Geometry check sheet. Reference: the model listing, model coordinates, mm. Coordinates: 2 decimals unless noted, no trailing zeros.
from build123d import *

# Parameters (mm, degrees)
F0_W           = 196.215
F0_H           = 38.1
F0_R           = 10.16
F0_R_2         = 6.604
F1_DEPTH       = 101.6
F2_D           = 12.7
F2_DEPTH       = 34.925
F2_CSINK_D     = 14.2875
F2_CSINK_ANGLE = 90
F2_TIP         = 3.8154649308
F3_ANGLE       = -90
F5_D           = 12.7
F5_DEPTH       = 34.925
F5_CSINK_D     = 14.2875
F5_CSINK_ANGLE = 90
F5_TIP         = 3.8154649308


with BuildPart() as f1:
    # F0 (on Top) → F1 (new body)
    with BuildSketch(Plane.XY):
        with Locations((849.6263678, -426.5737722)):
            Rectangle(F0_W, F0_H)
        with Locations((770.5688678, -426.5737722)):
            Circle(F0_R, mode=Mode.SUBTRACT)
        with Locations((849.6263678, -426.5737722)):
            Circle(F0_R, mode=Mode.SUBTRACT)
        with Locations((928.6838678, -426.5737722)):
            Circle(F0_R, mode=Mode.SUBTRACT)
        with Locations((770.5688678, -426.5737722)):
            Circle(F0_R)
        with Locations((770.5688678, -426.5737722)):
            Circle(F0_R_2, mode=Mode.SUBTRACT)
        with Locations((928.6838678, -426.5737722)):
            Circle(F0_R)
        with Locations((928.6838678, -426.5737722)):
            Circle(F0_R_2, mode=Mode.SUBTRACT)
        with Locations((849.6263678, -426.5737722)):
            Circle(F0_R)
        with Locations((849.6263678, -426.5737722)):
            Circle(F0_R_2, mode=Mode.SUBTRACT)
        with Locations((770.5688678, -426.5737722)):
            Circle(F0_R_2)
        with Locations((849.6263678, -426.5737722)):
            Circle(F0_R_2)
        with Locations((928.6838678, -426.5737722)):
            Circle(F0_R_2)
    extrude(amount=-F1_DEPTH)

    # F2
    with Locations(Plane.XY):
        with Locations((928.6838678, -426.5737722), (849.6263678, -426.5737722)):
            CounterSinkHole(F2_D / 2, F2_CSINK_D / 2, depth=F2_DEPTH, counter_sink_angle=F2_CSINK_ANGLE)
            with Locations((0, 0, -(F2_DEPTH + F2_TIP / 2))):  # 118° drill point
                Cone(0, F2_D / 2, F2_TIP, mode=Mode.SUBTRACT)


with BuildPart() as f1_1:
    # F3: moved
    add(f1.part.rotate(Axis((751.5188678, -426.5737722, 0), (0, -1, 0)), F3_ANGLE))


with BuildPart() as f1_2:
    # F4: moved
    add(f1_1.part.moved(Location((-50.8, 0, 0))))

    # F5
    with Locations(Plane.XY):
        with Locations((614.9938678, -426.5737722), (684.8438678, -426.5737722)):
            CounterSinkHole(F5_D / 2, F5_CSINK_D / 2, depth=F5_DEPTH, counter_sink_angle=F5_CSINK_ANGLE)
            with Locations((0, 0, -(F5_DEPTH + F5_TIP / 2))):  # 118° drill point
                Cone(0, F5_D / 2, F5_TIP, mode=Mode.SUBTRACT)


solid = f1_2.part
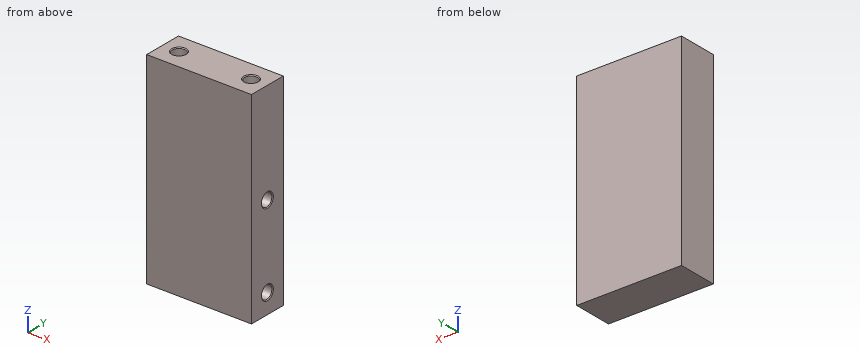
(1) Sectioned sample at A-A on x = 671.5. State how many separate pieces and enclosed holes the cut face has, and give its area (3 significant figures).
Findings:
separate pieces: 1
enclosed holes: 2
area: 7,220 mm2
(2) Gauge pin test, flat end, axial feed: pin 1 Ø7.5 at (x, y) = (614.99, -426.57) entering from +Z. Record the tip position at first contact, or that the pin passes through.
Findings:
pin 1: stops at z = -36.48
(3) Scan lines: L1, parallel to Z at x = 674, y = -424.5 (3 decimals); L2, parallel to Y at x = 693, z = -173.5; L3, parallel to Y at x = 610.5, z = -24.5. Record each from-to range of solid material in increasing order.
Findings:
L1: z = -196.215 to -183.167, -171.163 to -104.109, -92.106 to 0
L2: y = -445.62 to -431.76, -421.39 to -407.52
L3: y = -445.62 to -431.06, -422.09 to -407.52
